Read the model definition and answer for the solid it produces. Units are mm, in the model's axes. Face numbers are marked on the shaded views. A direction names the side the tool comes from. Coordinates: 2 decimals unless noted, no trailing zeros. Order: outer loops, then holes, each group sorted by start corner. A loop starts at its lowest first (then second) coordinate and runs counter-clockwise, first axis right, second up. Notation, with made-up numbers: (41.25, 11) -> (70.25, 11) arc R7 cw to (70.25, 19) -> close; hole circle Ø9 at (-31, 14). An arc over 180 degrees is marked (long way). Answer as a JSON object with one key per item and string values. Group by question number.
1) A tool of negligible diameter and unlimited length cuts with its end or side. For the marked faces 4 and 5, from which of +Z, -Z, +X, -X, +Y, -Y can it reach the whole face along a straight path? Write none if from no direction.
2) Consider L1, parallel to Z at x = 13, y = 0.4; L2, parallel to Z at x = 17.95, y = 30; L3, parallel to X at y = 37, z = 29.75. Determine where each line is inside the solid, lowest interval first.
3) Section A-A on y = 10.5 is taken. Determine the outline of the cut face in (x, z), and give its area (3 significant figures).
4) Section D-D on z = 34.5 is taken. Determine the outline of the cut face in (x, y), and give its area (3 significant figures).
5) Given pin 1 (1.5 mm diameter, centred on x = 13, z = 32, fed in from +Y); pin 2 (3 mm diameter, centred on x = 6, z = 32, fed in from +Y), each flat-ended and moving along its own axis, determine where each tip first touches the part or whether it passes through.
6) Determine the mould class of the marked faces 1, 2 and 3 for opening direction X: released by +X, released by -X, zero draft, split by the parting line, or undercut.
7) Section C-C on x = 13 is taken. Determine the outline of the cut face in (y, z).
8) Section B-B on z = 32 is taken. Determine the outline of the cut face in (x, y), and give its area (3 significant figures).
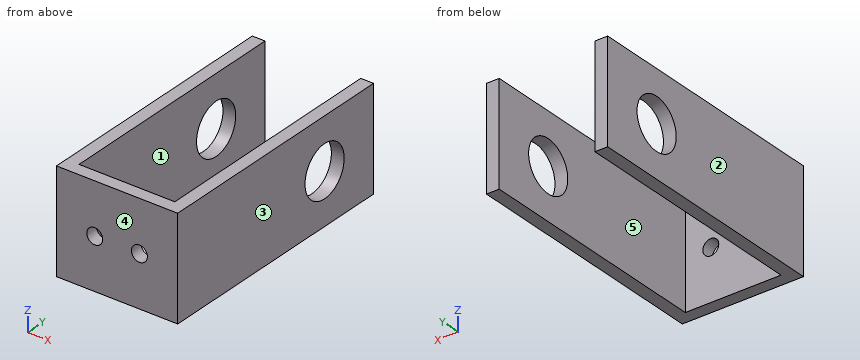
from build123d import *

# Parameters (mm, degrees)
EXTRUDE_1_DEPTH     = 40
SKETCH_2_R          = 4
CUT_EXTRUDE_1_DEPTH = 60.674114991
SKETCH_5_W          = 24
SKETCH_5_H          = 40
CUT_EXTRUDE_4_DEPTH = 60.674114991
SKETCH_6_R          = 1.25
CUT_EXTRUDE_5_DEPTH = 60.674114991


with BuildPart() as part:
    # 草图1 → 凸台-拉伸1 (new body)
    with BuildSketch(Plane.XY):
        Polygon((0, 0), (2, 0), (17, 0), (19, 0), (19, 40), (17, 40), (17, 2), (2, 2), (2, 40), (0, 40), align=None)
    extrude(amount=EXTRUDE_1_DEPTH)

    # 草图2 → 切除-拉伸1 (cut, through all)
    with BuildSketch(Plane(origin=(19, 0, 0), x_dir=(0, 0, -1), z_dir=(1, 0, 0))):
        with Locations(Location((-32, 30, 0), (0, 0, 90))):
            Circle(SKETCH_2_R)
    extrude(amount=-CUT_EXTRUDE_1_DEPTH, mode=Mode.SUBTRACT)

    # 草图5 → 切除-拉伸4 (cut, through all)
    with BuildSketch(Plane.ZY):
        with Locations((12, 20)):
            Rectangle(SKETCH_5_W, SKETCH_5_H)
    extrude(amount=-CUT_EXTRUDE_4_DEPTH, mode=Mode.SUBTRACT)

    # 草图6 → 切除-拉伸5 (cut, through all)
    with BuildSketch(Plane.XZ):
        with Locations((13, 32)):
            Circle(SKETCH_6_R)
        with Locations(Location((6, 32, 0), (0, 0, 270))):
            Circle(SKETCH_6_R)
    extrude(amount=-CUT_EXTRUDE_5_DEPTH, mode=Mode.SUBTRACT)


solid = part.part
Worked answers:
{
 "1": {"face 4": "+Z, -Z, +X, -X, -Y", "face 5": "+Z, -Z, +Y"},
 "2": {"L1": "z = 24 to 30.75, 33.25 to 40", "L2": "z = 24 to 28, 36 to 40", "L3": "x = 0 to 2, 17 to 19"},
 "3": {"outline": "(0, 24) -> (2, 24) -> (2, 40) -> (0, 40) -> close; (17, 24) -> (19, 24) -> (19, 40) -> (17, 40) -> close", "area": "64.0 mm²"},
 "4": {"outline": "(0, 0) -> (19, 0) -> (19, 26.88) -> (17, 26.88) -> (17, 2) -> (2, 2) -> (2, 26.88) -> (0, 26.88) -> close; (0, 33.12) -> (2, 33.12) -> (2, 40) -> (0, 40) -> close; (17, 33.12) -> (19, 33.12) -> (19, 40) -> (17, 40) -> close", "area": "165 mm²"},
 "5": {"pin 1": "passes through", "pin 2": "stops at y = 2"},
 "6": {"face 1": "undercut", "face 2": "released by -X", "face 3": "released by +X"},
 "7": {"outline": "(0, 24) -> (2, 24) -> (2, 30.75) -> (0, 30.75) -> close; (0, 33.25) -> (2, 33.25) -> (2, 40) -> (0, 40) -> close"},
 "8": {"outline": "(0, 0) -> (4.75, 0) -> (4.75, 2) -> (2, 2) -> (2, 26) -> (0, 26) -> close; (0, 34) -> (2, 34) -> (2, 40) -> (0, 40) -> close; (7.25, 0) -> (11.75, 0) -> (11.75, 2) -> (7.25, 2) -> close; (14.25, 0) -> (19, 0) -> (19, 26) -> (17, 26) -> (17, 2) -> (14.25, 2) -> close; (17, 34) -> (19, 34) -> (19, 40) -> (17, 40) -> close", "area": "148 mm²"}
}
